Source: CAD feature listing. Evaluate the final solid. Frame: model axes, mm. A direction names the side the tool comes from. Round coordinates to 2 decimals unless told otherwise and drop trailing zeros. One line per item, written item: value. Start each with the question number.
1) Ray query, L1, parallel to X at y = 2.5, z = 32; L2, parallel to X at y = 4.7, z = 9.5. Return the intervals inside material, ascending.
2) Mould query, pull axis X, two halves, no side actions, for faces 1 (the face through (27.576, 0.811, 31.227)), 2 (the face through (8, 4.9, 24)). Classes: pulls with the +X half, pulls with the -X half, needs draft (parallel to the pull), parting line crosses it, or undercut.
3) Pin query (flat end, axial travel): P1, Ø1.4, axis at x = 28.5, z = 28, coming from the -Y side; P2, Ø2, axis at x = 13, z = 18, coming from the +Y side; P3, Ø0.8, axis at x = 0, z = 24, coming from the -Y side. Return the tip coordinate at first contact, or that it passes through.
4) Section A-A (y = 3.8). State how many separate pieces and enclosed holes the cut face has, and give its area (3 significant figures).
5) Reachability of faces 3 (the face through (5.29, 0.811, 6.024)), 4 (the face through (0, 4.9, 8)), 5 (the face through (1.29, 4.038, -2.024)) from +Z, -Z, +X, -X, +Y, -Y: full face, straight path, thin tool, end or side. Return the list, or none.
```python
from build123d import *

# Parameters (mm, degrees)
SKETCH_1_W                  = 8
SKETCH_1_H                  = 8
HEIGHT_DEPTH                = 3.2
SKETCH_2_R                  = 2.4
EXTRUDE_2_DEPTH             = 1.7
PATTERN_LINEAR_1_COUNT      = 5
PATTERN_LINEAR_1_PITCH      = 8
PATTERN_LINEAR_1_COUNT_DIR2 = 5
PATTERN_LINEAR_1_PITCH_DIR2 = 8
SHELL_1_T                   = -1.6
SKETCH_3_R                  = 3.255
SKETCH_3_R_2                = 2.4
EXTRUDE_3_DEPTH             = 1.6
PATTERN_LINEAR_2_COUNT      = 4
PATTERN_LINEAR_2_PITCH      = 8
PATTERN_LINEAR_2_COUNT_DIR2 = 4
PATTERN_LINEAR_2_PITCH_DIR2 = 8


with BuildPart() as part:
    # 草圖1 → height (new body)
    with BuildSketch(Plane(origin=(0, 0, 0), x_dir=(1, 0, 0), z_dir=(0, 1, 0))):
        Rectangle(SKETCH_1_W, SKETCH_1_H)
    height = extrude(amount=HEIGHT_DEPTH)

    # 草圖2 → 填料-伸長2 (add)
    with BuildSketch(Plane(origin=(0, 3.2, 0), x_dir=(1, 0, 0), z_dir=(0, 1, 0))):
        Circle(SKETCH_2_R)
    extrude_2 = extrude(amount=EXTRUDE_2_DEPTH)

    # 直線複製排列1: height, Extrude 2 5 × 5
    with Locations(*[(i * PATTERN_LINEAR_1_PITCH, 0, j * PATTERN_LINEAR_1_PITCH_DIR2) for i in range(PATTERN_LINEAR_1_COUNT) for j in range(PATTERN_LINEAR_1_COUNT_DIR2) if (i, j) != (0, 0)]):
        add(height)
        add(extrude_2)

    # 薄殼1
    shell_1_openings = [part.faces().sort_by_distance(p)[0] for p in [
        (16, 0, 16),
    ]]
    offset(amount=SHELL_1_T, openings=shell_1_openings, kind=Kind.INTERSECTION)

    # 草圖3 → 填料-伸長3 (add)
    with BuildSketch(Plane.XZ.offset(-1.6)):
        with Locations((4, 4)):
            Circle(SKETCH_3_R)
        with Locations((4, 4)):
            Circle(SKETCH_3_R_2, mode=Mode.SUBTRACT)
    extrude_3 = extrude(amount=EXTRUDE_3_DEPTH)

    # 直線複製排列2: Extrude 3 4 × 4
    with Locations(*[(j * PATTERN_LINEAR_2_PITCH_DIR2, 0, i * PATTERN_LINEAR_2_PITCH) for i in range(PATTERN_LINEAR_2_COUNT) for j in range(PATTERN_LINEAR_2_COUNT_DIR2) if (i, j) != (0, 0)]):
        add(extrude_3)


solid = part.part
```
Findings:
1. L1: -4 to -0.8, 0.8 to 7.2, 8.8 to 15.2, 16.8 to 23.2, 24.8 to 31.2, 32.8 to 36
1. L2: -1.87 to 1.87, 6.13 to 9.87, 14.13 to 17.87, 22.13 to 25.87, 30.13 to 33.87
2. face 1: undercut
2. face 2: needs draft
3. P1: y = 1.6
3. P2: y = 3.2
3. P3: y = 3.3
4. separate pieces: 25
4. enclosed holes: 0
4. area: 452 mm2
5. face 3: -Y
5. face 4: +Z, -Z, +X, -X, +Y
5. face 5: +Y
